Geometry check sheet. Reference: the model listing, model coordinates, mm. Face numbers are marked on the shaded views. A direction names the side the tool comes from. Give positions to 0.01 mm unless a question says otherwise; leave off trailing zeros. Order: outer loops, then holes, each group sorted by start corner. A loop starts at its lowest first (then second) coordinate and runs counter-clockwise, first axis right, second up. Notation, with made-up numbers: M 42.25,27 L 69.25,27 A21 cw 69.25,40 Z; hole C 80.5,30.5 d11. An arc over 180 degrees is marked long. Use CSV: the item, a comma, the result in double quotes. Start each with the question number.
from build123d import *

# Parameters (mm, degrees)
F0_R     = 39
F0_R_2   = 37.5
F1_DEPTH = 13
F2_R     = 40
F2_R_2   = 37.5
F3_DEPTH = 1.5


with BuildPart() as f1:
    # F0 (on Top) → F1 (new body)
    with BuildSketch(Plane.XY):
        Circle(F0_R)
        Circle(F0_R_2, mode=Mode.SUBTRACT)
    extrude(amount=F1_DEPTH)

    # F2 (on Top) → F3 (join, symmetric)
    with BuildSketch(Plane.XY):
        Circle(F2_R)
        Circle(F2_R_2, mode=Mode.SUBTRACT)
    extrude(amount=F3_DEPTH, both=True)

    # F4 (on Right) → F5 (revolve)
    with BuildSketch(Plane.YZ):
        Polygon((39.990474, -2.075957), (40.046833, 0), (32.043573, 0), (16.581262, -6.303032), (0, -6.303032), (0, -8.613833), (16.571351, -8.613833), (32.719906, -2.075957), align=None)
    revolve(axis=Axis((0, 0, -7.458432), (0, 0, -1)))


solid = f1.part
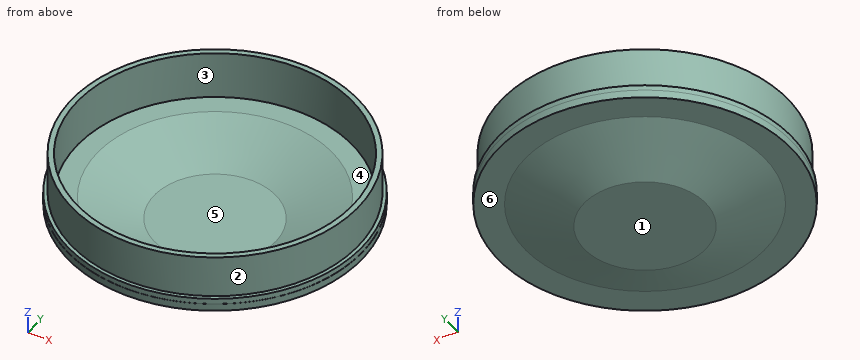
(1) Thickness scan on line 1 (X direction, y = 0, z = 5.5); line 2 (Z direction, x = 25, y = -23.5). Record the ranges inside material, lowest first.
(2) Go/stop test with flat-tipped pins: P1, Ø8, axis at x = -27, z = 10, coming from the -Y side; P2, Ø24, axis at x = 10, y = 10.5, coming from the +Z side; P3, Ø3, axis at x = -9.5, y = 21, coming from the -Z side. Record where each tip stops, or that it passes through.
(3) Draft check along X on the marked faces 1, 2, 3 and 4. Enter one of: +X half, -X half, draft (parallel to the pull), parting line (faces both ways), or undercut.
(4) Sectioned sample at A-A on x = 0. Record the cut outline in (y, z), then the cut area to 3 significant figures.
(5) Sectioned sample at C-C on z = 6.75. Record the cut outline in (x, y), then the cut area to 3 significant figures.
(6) Access from +Z, -Z, +X, -X, +Y, -Y to the whole of each face (thin tool, end or side, straight path). Record for the marked faces 5 and 6.
Responses:
1,line 1,"-39 to -37.5, 37.5 to 39"
1,line 2,"-2.08 to 0"
2,P1,"y = -31.5"
2,P2,"z = -2.26"
2,P3,"z = -6.6"
3,face 1,"draft"
3,face 2,"parting line"
3,face 3,"undercut"
3,face 4,"undercut"
4,outline,"M -40.05,0 L -39.99,-2.08 L -32.72,-2.08 L -16.57,-8.61 L 16.57,-8.61 L 32.72,-2.08 L 39.99,-2.08 L 40.05,0 L 40,0 L 40,1.5 L 39,1.5 L 39,13 L 37.5,13 L 37.5,0 L 32.04,0 L 16.58,-6.3 L -16.58,-6.3 L -32.04,0 L -37.5,0 L -37.5,13 L -39,13 L -39,1.5 L -40,1.5 L -40,0 Z"
4,area,"224 mm2"
5,outline,"C 0,0 d78; hole C 0,0 d75"
5,area,"360 mm2"
6,face 5,"+Z"
6,face 6,"-Z"
